```python
from build123d import *

# Parameters (mm, degrees)
SKETCH1_R               = 1.5
BOSS_EXTRUDE1_DEPTH     = 3
SKETCH2_R               = 1.5
CUT_EXTRUDE1_DEPTH      = 53.82281704
BOSS_EXTRUDE2_START     = -3
SKETCH3_R               = 1.5
BOSS_EXTRUDE2_DEPTH     = 3
BOSS_EXTRUDE3_START     = -16.5
BOSS_EXTRUDE3_OUTLINE_W = 3
BOSS_EXTRUDE3_OUTLINE_H = 47
BOSS_EXTRUDE3_DEPTH     = 13.5
BOSS_EXTRUDE5_DEPTH     = 3
CUT_EXTRUDE2_DEPTH      = 103.691284927
BOSS_EXTRUDE6_DEPTH     = 3
CUT_EXTRUDE3_DEPTH      = 103.691284927


# Read off the part's stored shape, not the designer's step: Boss-Extrude3
with BuildPart() as part:
    # Sketch1 → Boss-Extrude1 (new body)
    with BuildSketch(Plane(origin=(0, 0, 0), x_dir=(1, 0, 0), z_dir=(0, 1, 0))):
        with BuildLine():
            Line((37, 27.5), (-37, 27.5))
            ThreePointArc((-37, 27.5), (-42.656854249, 25.156854249), (-45, 19.5))
            Line((-45, 19.5), (-45, -19.5))
            ThreePointArc((-45, -19.5), (-42.656854249, -25.156854249), (-37, -27.5))
            Line((-37, -27.5), (37, -27.5))
            ThreePointArc((37, -27.5), (42.656854249, -25.156854249), (45, -19.5))
            Line((45, -19.5), (45, 19.5))
            ThreePointArc((45, 19.5), (42.656854249, 25.156854249), (37, 27.5))
        make_face()
        with Locations(Location((-22.790794979, 24.5, 0), (0, 0, 270))):
            Circle(SKETCH1_R, mode=Mode.SUBTRACT)
        with Locations(Location((-22.790794979, -24.5, 0), (0, 0, 270))):
            Circle(SKETCH1_R, mode=Mode.SUBTRACT)
        with Locations(Location((35.209205021, -24.5, 0), (0, 0, 270))):
            Circle(SKETCH1_R, mode=Mode.SUBTRACT)
        with Locations(Location((35.209205021, 24.5, 0), (0, 0, 270))):
            Circle(SKETCH1_R, mode=Mode.SUBTRACT)
        with Locations(Location((-40.029839799, 10, 0), (0, 0, 270))):
            Circle(SKETCH1_R, mode=Mode.SUBTRACT)
        with Locations(Location((-40.029839799, -10, 0), (0, 0, 270))):
            Circle(SKETCH1_R, mode=Mode.SUBTRACT)
    extrude(amount=BOSS_EXTRUDE1_DEPTH)

    # Sketch2 → Cut-Extrude1 (cut, through all)
    with BuildSketch(Plane(origin=(0, 3, 0), x_dir=(1, 0, 0), z_dir=(0, 1, 0))):
        with Locations(Location((23.470160201, 10, 0), (0, 0, 270))):
            Circle(SKETCH2_R)
        with Locations(Location((23.470160201, -10, 0), (0, 0, 270))):
            Circle(SKETCH2_R)
    extrude(amount=-CUT_EXTRUDE1_DEPTH, mode=Mode.SUBTRACT)

    # Sketch3 → Boss-Extrude2 (add)
    with BuildSketch(Plane(origin=(0, 3, 0), x_dir=(1, 0, 0), z_dir=(0, 1, 0)).offset(BOSS_EXTRUDE2_START)):
        with BuildLine():
            Line((-37, 27.5), (-87, 27.5))
            ThreePointArc((-87, 27.5), (-94.071067812, 24.571067812), (-97, 17.5))
            Line((-97, 17.5), (-97, -17.5))
            ThreePointArc((-97, -17.5), (-94.071067812, -24.571067812), (-87, -27.5))
            Line((-87, -27.5), (-37, -27.5))
            Line((-37, -27.5), (-37, 27.5))
        make_face()
        with Locations(Location((-40.029839799, 10, 0), (0, 0, 270))):
            Circle(SKETCH3_R, mode=Mode.SUBTRACT)
        with Locations(Location((-40.029839799, -10, 0), (0, 0, 270))):
            Circle(SKETCH3_R, mode=Mode.SUBTRACT)
    extrude(amount=BOSS_EXTRUDE2_DEPTH)

    # Boss-Extrude3 outline → Boss-Extrude3 (add)
    with BuildSketch(Plane(origin=(0, 3, 0), x_dir=(1, 0, 0), z_dir=(0, 1, 0)).offset(BOSS_EXTRUDE3_START)):
        with BuildLine():
            Line((-97, 17.5), (-97, -17.5))
            ThreePointArc((-97, -17.5), (-96.486832981, -20.66227766), (-95, -23.5))
            Line((-95, -23.5), (-94.029839799, -23.5))
            Line((-94.029839799, -23.5), (-94.029839799, 23.5))
            Line((-94.029839799, 23.5), (-95, 23.5))
            ThreePointArc((-95, 23.5), (-96.486832981, 20.66227766), (-97, 17.5))
        make_face()
        with Locations((-45.529839799, 0)):
            Rectangle(BOSS_EXTRUDE3_OUTLINE_W, BOSS_EXTRUDE3_OUTLINE_H)
    extrude(amount=BOSS_EXTRUDE3_DEPTH)

    # Sketch6 → Boss-Extrude5 (add)
    with BuildSketch(Plane.XZ.offset(13.5)):
        with BuildLine():
            Line((-44.029839799, 23.5), (-46.029839799, 23.5))
            ThreePointArc((-46.029839799, 23.5), (-53.100907611, 20.571067812), (-56.029839799, 13.5))
            Line((-56.029839799, 13.5), (-56.029839799, -13.5))
            ThreePointArc((-56.029839799, -13.5), (-53.100907611, -20.571067812), (-46.029839799, -23.5))
            Line((-46.029839799, -23.5), (-44.029839799, -23.5))
            Line((-44.029839799, -23.5), (-44.029839799, 23.5))
        make_face()
        with BuildLine():
            Line((-85.136084996, -13.5), (-85.136084996, 13.5))
            ThreePointArc((-85.136084996, 13.5), (-88.065017184, 20.571067812), (-95.136084996, 23.5))
            Line((-95.136084996, 23.5), (-97, 23.5))
            Line((-97, 23.5), (-97, -23.5))
            Line((-97, -23.5), (-95.136084996, -23.5))
            ThreePointArc((-95.136084996, -23.5), (-88.065017184, -20.571067812), (-85.136084996, -13.5))
        make_face()
    extrude(amount=BOSS_EXTRUDE5_DEPTH)

    # Sketch7 → Cut-Extrude2 (cut, through all)
    with BuildSketch(Plane(origin=(0, 3, 0), x_dir=(1, 0, 0), z_dir=(0, 1, 0))):
        with BuildLine():
            Line((-97, 27.5), (-87, 27.5))
            ThreePointArc((-87, 27.5), (-94.071067812, 24.571067812), (-97, 17.5))
            Line((-97, 17.5), (-97, 27.5))
        make_face()
        with BuildLine():
            Line((-97, -27.5), (-97, -17.5))
            ThreePointArc((-97, -17.5), (-94.071067812, -24.571067812), (-87, -27.5))
            Line((-87, -27.5), (-97, -27.5))
        make_face()
    extrude(amount=-CUT_EXTRUDE2_DEPTH, mode=Mode.SUBTRACT)

    # Sketch8 → Boss-Extrude6 (add)
    with BuildSketch(Plane.XY.offset(23.5)):
        with BuildLine():
            Line((-50.029839799, -16.5), (-46.029839799, -16.5))
            Line((-46.029839799, -16.5), (-46.029839799, -13.5))
            Line((-46.029839799, -13.5), (-47.029839799, -13.5))
            Line((-47.029839799, -13.5), (-47.029839799, -6.75))
            Line((-47.029839799, -6.75), (-56.029839799, -6.75))
            Line((-56.029839799, -6.75), (-56.029839799, -10.5))
            ThreePointArc((-56.029839799, -10.5), (-54.272480486, -14.742640687), (-50.029839799, -16.5))
        make_face()
        with BuildLine():
            Line((-47.029839799, -6.75), (-47.029839799, 0))
            Line((-47.029839799, 0), (-50.029839799, 0))
            ThreePointArc((-50.029839799, 0), (-54.272480486, -1.757359313), (-56.029839799, -6))
            Line((-56.029839799, -6), (-56.029839799, -6.75))
            Line((-56.029839799, -6.75), (-47.029839799, -6.75))
        make_face()
        Polygon((-44.029839799, -16.5), (-44.029839799, 0), (-47.029839799, 0), (-47.029839799, -13.5), (-46.029839799, -13.5), (-46.029839799, -16.5), align=None)
        with BuildLine():
            Line((-95, -6.75), (-85.136084996, -6.75))
            Line((-85.136084996, -6.75), (-85.136084996, -6))
            ThreePointArc((-85.136084996, -6), (-86.893444309, -1.757359313), (-91.136084996, 0))
            Line((-91.136084996, 0), (-95, 0))
            Line((-95, 0), (-95, -6.75))
        make_face()
        with BuildLine():
            Line((-85.136084996, -10.493579037), (-85.136084996, -6.75))
            Line((-85.136084996, -6.75), (-95, -6.75))
            Line((-95, -6.75), (-95, -16.48944967))
            Line((-95, -16.48944967), (-91.142502523, -16.493575605))
            ThreePointArc((-91.142502523, -16.493575605), (-86.895713854, -14.738488056), (-85.136084996, -10.493579037))
        make_face()
    extrude(amount=BOSS_EXTRUDE6_DEPTH)

    # Sketch9 → Cut-Extrude3 (cut, through all)
    with BuildSketch(Plane(origin=(0, 3, 0), x_dir=(1, 0, 0), z_dir=(0, 1, 0))):
        with BuildLine():
            Line((-97, -17.5), (-97, -27.5))
            Line((-97, -27.5), (-87, -27.5))
            ThreePointArc((-87, -27.5), (-94.071067812, -24.571067812), (-97, -17.5))
        make_face()
    extrude(amount=-CUT_EXTRUDE3_DEPTH, mode=Mode.SUBTRACT)


solid = part.part
```
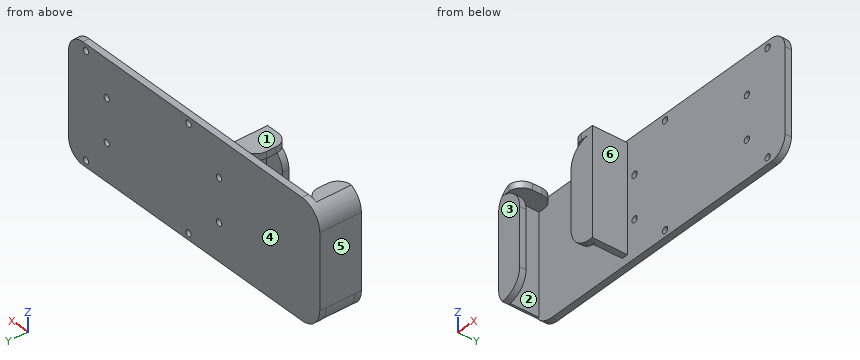
Geometry check sheet. Reference: the model listing, model coordinates, mm. Face numbers are marked on the shaded views. A direction names the side the tool comes from. Coordinates: 2 decimals unless noted, no trailing zeros. Order: outer loops, then holes, each group sorted by start corner. A loop starts at its lowest first (then second) coordinate and runs counter-clockwise, first axis right, second up. Notation, with made-up numbers: (35, -38.75) - (71, -38.75) arc R20 cw to (71, -27.75) - close; hole circle Ø7 at (14, 49). An arc over 180 degrees is marked (long way). Answer as a JSON object with one key per item and string values. Group by question number.
Item 1: Sectioned sample at A-A, the plane y = -9. Record the cut outline in (x, z), and give its area (3 significant figures).
Item 2: Tool access check on the marked faces 5 and 6. Record the directions out of +Z, -Z, +X, -X, +Y, -Y that give a thin tool (end or side, any length) a straight path to the whole face; none if there is none.
Item 3: Sectioned sample at D-D, the plane y = 1.25. Give the number of separate pieces and of enclosed holes in the cut face, and give its area (3 significant figures).
Item 4: Sectioned sample at B-B, the plane z = -10. Record the cut outline in (x, y).
Item 5: Sectioned sample at C-C, the plane z = -3.5. Record the cut outline in (x, y).
Item 6: Scan lines: probe 1 along X at (y, z) = (1.75, -10); probe 2 along X at (y, z) = (-7.25, 13.5); probe 3 along X at (y, z) = (0.85, -24.5) (3 decimals). Record each from-to range of solid material in increasing order.
Item 7: Draft check along Y on the marked faces 1, 2, 3 and 4. Enter one of: +Y half, -Y half, draft (parallel to the pull), parting line (faces both ways), or undercut.
Item 8: Depth check by flat-ended pin: pin 1 Ø4 at (y, z) = (-2, -21.5) entering from -X; pin 2 Ø7 at (x, y) = (-88, -6) entering from +Z; pin 3 Ø4 at (y, z) = (-10, 1.5) entering from +X; pin 4 Ø2.5 at (x, z) = (-22.79, 24.5) entering from -Y. Enter the tip coordinate at first touch or a pass-through.
Resolved:
{
 "1": {"outline": "(-97, -17.5) arc R10 ccw to (-95, -23.5) - (-94.03, -23.5) - (-94.03, 23.5) - (-85.14, 23.5) - (-85.14, 26.5) - (-91.36, 26.5) arc R10 ccw to (-97, 17.5) - close; (-56.03, 23.5) - (-47.03, 23.5) - (-47.03, -23.5) - (-44.03, -23.5) - (-44.03, 26.5) - (-56.03, 26.5) - close", "area": "334 mm^2"},
 "2": {"face 5": "+Z, -Z, -X, +Y, -Y", "face 6": "+Z, -Z, +X, -Y"},
 "3": {"separate pieces": "1", "enclosed holes": "8", "area": "7,680 mm^2"},
 "4": {"outline": "(-97, -16.5) - (-85.14, -16.5) - (-85.14, -13.5) - (-94.03, -13.5) - (-94.03, 0) - (-47.03, 0) - (-47.03, -13.5) - (-56.03, -13.5) - (-56.03, -16.5) - (-44.03, -16.5) - (-44.03, 0) - (-41.53, 0) - (-41.53, 3) - (-97, 3) - close; (-38.53, 0) - (21.97, 0) - (21.97, 3) - (-38.53, 3) - close; (24.97, 0) - (45, 0) - (45, 3) - (24.97, 3) - close"},
 "5": {"outline": "(-97, -16.5) - (-85.14, -16.5) - (-85.14, -13.5) - (-94.03, -13.5) - (-94.03, 0) - (-47.03, 0) - (-47.03, -13.5) - (-56.03, -13.5) - (-56.03, -16.5) - (-44.03, -16.5) - (-44.03, 0) - (45, 0) - (45, 3) - (-97, 3) - close"},
 "6": {"probe 1": "-97 to -41.53, -38.53 to 21.97, 24.97 to 45", "probe 2": "-97 to -94.03, -47.03 to -44.03", "probe 3": "-94.141 to -24.291, -21.291 to 33.709, 36.709 to 43.245"},
 "7": {"face 1": "draft", "face 2": "undercut", "face 3": "-Y half", "face 4": "+Y half"},
 "8": {"pin 1": "x = -96.8", "pin 2": "z = 26.5", "pin 3": "x = -44.03", "pin 4": "through"}
}
